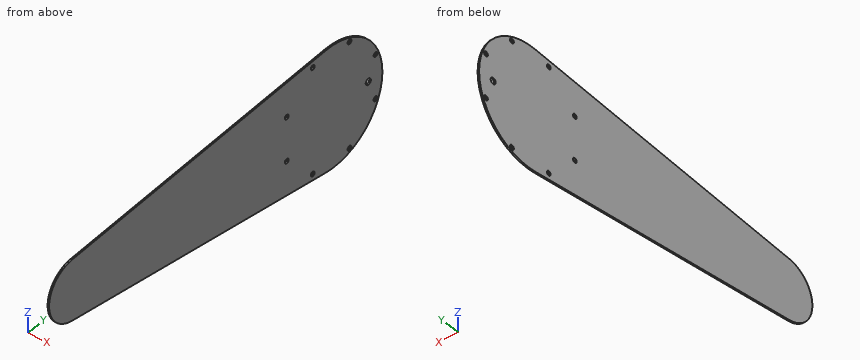
Autodesk Inventor part; units mm, degrees
ref_plane "YZ Plane" through (0, 0, 0) normal (1, 0, 0) x (0, 1, 0)
ref_plane "XZ Plane" through (0, 0, 0) normal (0, 1, 0) x (-1, 0, 0)
ref_plane "XY Plane" through (0, 0, 0) normal (0, 0, 1) x (1, 0, 0)
sketch "スケッチ1" plane through (0, 0, 0) normal (1, 0, 0) x (0, 1, 0)
  circle A0 centre (0, 0) radius 40
  dimension "d0" = 80
extrude "押し出し1" add sketch "スケッチ1" along normal blind 1
sketch "スケッチ2" plane through (1, 0, 0) normal (1, 0, 0) x (0, 0, -1)
  point P0 (0, 0)
  point P1 (0, 29)
  dimension "d3" = 29
hole "穴1" at (1, 29, 0) direction (-1, 0, 0) diameter 4 end through all
sketch "スケッチ4" plane through (1, 0, 0) normal (1, 0, 0) x (0, 0, -1)
  circle A0 centre (0, -200) radius 20
  circle A1 centre (0, 0) radius 40
  line L0 (-39.7995, -4) -> (-19.8997, -202)
  line L1 (39.7995, -4) -> (19.8997, -202)
  circle A2 centre (0, 0) radius 40
  dimension "d13" = 40
  dimension "d14" = 200
extrude "押し出し2" add sketch "スケッチ4" against normal blind 1 contours A0 | A0 L0 A1 L1
sketch "スケッチ5" plane through (0, 0, 0) normal (-1, 0, 0) x (0, 0, 1)
  line L0 (-14.3506, 34.6455) -> (14.3506, 34.6455)
  line L1 (14.3506, 34.6455) -> (34.6455, 14.3506)
  line L2 (34.6455, 14.3506) -> (34.6455, -14.3506)
  line L3 (34.6455, -14.3506) -> (14.3506, -34.6455)
  line L4 (14.3506, -34.6455) -> (-14.3506, -34.6455)
  line L5 (-14.3506, -34.6455) -> (-34.6455, -14.3506)
  line L6 (-34.6455, -14.3506) -> (-34.6455, 14.3506)
  line L7 (-34.6455, 14.3506) -> (-14.3506, 34.6455)
  circle A0 centre (0, 29) radius 2
  line L8 (0, 0) -> (0, 29)
  dimension "d17" = 37.5
hole "穴2" at (0, 34.6455, -14.3506) at (0, 14.3506, -34.6455) at (0, -14.3506, -34.6455) at (0, -34.6455, -14.3506) at (0, -34.6455, 14.3506) at (0, -14.3506, 34.6455) at (0, 14.3506, 34.6455) at (0, 34.6455, 14.3506) direction (1, 0, 0) diameter 3 end through all
properties part number "main_plate"
Geometry check sheet. Reference: the model listing, model coordinates, mm. Give positions to 0.01 mm unless a question says otherwise; leave off trailing zeros. Order: outer loops, then holes, each group sorted by start corner. A loop starts at its lowest first (then second) coordinate and runs counter-clockwise, first axis right, second up. Notation, with made-up numbers: (41, 33.25) - (81, 33.25) arc R16 ccw to (81, 64.25) - close; hole circle Ø8 at (3.25, -2). An arc over 180 degrees is marked (long way). Answer as a JSON object with one key per item and string values.
(1) Cross-section at B-B (y = 21). Record the cut outline in (x, z), then the cut area to 3 significant figures.
Report:
{"outline": "(0, -34.04) - (1, -34.04) - (1, 34.04) - (0, 34.04) - close", "area": "68.1 mm^2"}
(2) Depth check by flat-ended pin: pin 1 Ø1.8 at (y, z) = (-14.35, -34.65) entering from -X. Enter the tip coordinate at first touch or a pass-through.
Report:
{"pin 1": "through"}
(3) Cross-section at C-C (z = -26). Record the cut outline in (x, y).
Report:
{"outline": "(0, -141.3) - (1, -141.3) - (1, 30.4) - (0, 30.4) - close"}
(4) Material ranges on line 1 (Y direction, x = 0.3, z = -15); line 2 (Z direction, x = 0.35, y = 28); line 3 (Y direction, x = 0.4, z = 16), recorded low to high.
Report:
{"line 1": "-213.23 to -36, -33.29 to 33.29, 36 to 37.08", "line 2": "-28.57 to -1.73, 1.73 to 28.57", "line 3": "-212 to 36.66"}
(5) Cross-section at A-A (x = 0.4). State how many separate pieces and enclosed holes the cut face has, then the cut area to 3 significant figures.
Report:
{"separate pieces": "1", "enclosed holes": "9", "area": "15,100 mm^2"}
